Autodesk Inventor part; units mm, degrees
ref_plane "YZ Plane" through (0, 0, 0) normal (1, 0, 0) x (0, 1, 0)
ref_plane "XZ Plane" through (0, 0, 0) normal (0, 1, 0) x (-1, 0, 0)
ref_plane "XY Plane" through (0, 0, 0) normal (0, 0, 1) x (1, 0, 0)
sketch "Sketch1" plane through (0, 0, 0) normal (0, 1, 0) x (-1, 0, 0)
  line L0 (0, 0) -> (8.75, 0) construction
  circle A0 centre (8.75, 0) radius 1.75
  circle A1 centre (8.75, 0) radius 2.5
  line L1 (0, 0) -> (-8.75, 0) construction
  circle A2 centre (-8.75, 0) radius 1.75
  circle A3 centre (-8.75, 0) radius 2.5
  line L2 (8.75, 2.5) -> (-8.75, 2.5)
  line L3 (8.75, -2.5) -> (-8.75, -2.5)
  dimension "d0" = 8.75
  dimension "d1" = 3.5
  dimension "d2" = 5
  dimension "d3" = 8.75
  dimension "d4" = 3.5
  dimension "d5" = 5
extrude "Extrusion1" add sketch "Sketch1" along normal blind 2.5
sketch "Sketch2" plane through (0, 2.5, 0) normal (0, 1, 0) x (1, 0, 0)
  circle A0 centre (8.75, 0) radius 1.75
  circle A1 centre (8.75, 0) radius 2.5
  point P0 (0, 0)
  dimension "d8" = 5
extrude "Extrusion2" add sketch "Sketch2" along normal blind 2.5
properties part number "eje de servo 2"
Source: CAD feature listing. Evaluate the final solid. Frame: model axes, mm. Coordinates: 2 decimals unless noted, no trailing zeros. Loops run counter-clockwise (first coordinate to the right, second up) from the corner with the lowest first, then second, coordinate; pieces in that order, holes last. Notation, with made-up numbers: (44.25, 21.5) - (68.25, 21.5) arc R10 ccw to (68.25, 33.5) - close; hole circle Ø6 at (35, -27). An arc over 180 degrees is marked (long way). Answer as CSV lines item,"result".
1. Mould query, pull axis Z, two halves, no side actions, for faces 1 (the cylindrical face through (10.954, 2.465, -1.179)), 2 (the cylindrical face through (8.635, 2.465, -1.746)), 3 (the flat face through (-1, 2.5, 0)). Classes: released by +Z, released by -Z, zero draft, split by the parting line, or undercut.
Established:
face 1,"split by the parting line"
face 2,"undercut"
face 3,"zero draft"
2. Ray query, line 1 (X direction, y = 3.65, z = 0); line 2 (X direction, y = 0.7, z = -0.15); line 3 (Z direction, x = -8.75, y = 1). Return the intervals inside material, ascending.
Established:
line 1,"x = 6.25 to 7, 10.5 to 11.25"
line 2,"x = -11.25 to -10.49, -7.01 to 7.01, 10.49 to 11.25"
line 3,"z = -2.5 to -1.75, 1.75 to 2.5"
3. Section D-D (y = 4.6). Return loops of the section in (x, z).
Established:
outline,"circle Ø5 at (8.75, 0); hole circle Ø3.5 at (8.75, 0)"
4. Contact query for flat-ended pins moving along their axis: pin 1 (1 mm diameter, centred on x = -1.5, z = 0, fed in from +Y); pin 2 (3 mm diameter, centred on y = 4.5, z = -1, fed in from +X); pin 3 (3 mm diameter, centred on x = 8.75, z = 0, fed in from +Y). Output: stop coordinate, or through.
Established:
pin 1,"stops at y = 2.5"
pin 2,"stops at x = 11.25"
pin 3,"passes through"
5. Section A-A (z = 0.6). Return loops of the section in (x, y).
Established:
outline,"(-11.18, 0) - (-10.39, 0) - (-10.39, 2.5) - (-11.18, 2.5) - close; (-7.11, 0) - (7.11, 0) - (7.11, 5) - (6.32, 5) - (6.32, 2.5) - (-7.11, 2.5) - close; (10.39, 0) - (11.18, 0) - (11.18, 5) - (10.39, 5) - close"
6. Section B-B (y = 0.85). Return loops of the section in (x, z), then the cut area to 3 significant figures.
Established:
outline,"(-8.75, -2.5) - (8.75, -2.5) arc R2.5 ccw to (8.75, 2.5) - (-8.75, 2.5) arc R2.5 ccw to start; hole circle Ø3.5 at (-8.75, 0); hole circle Ø3.5 at (8.75, 0)"
area,"87.9 mm2"
